Part model, mm, in its own coordinate system. A direction names the side the tool comes from. Coordinates: 2 decimals unless noted, no trailing zeros. Loops run counter-clockwise (first coordinate to the right, second up) from the corner with the lowest first, then second, coordinate; pieces in that order, holes last. Notation, with made-up numbers: (-20.75, 55.25) - (4.25, 55.25) arc R10 cw to (4.25, 71.25) - close; hole circle Ø8 at (34.25, 40.5). An arc over 180 degrees is marked (long way). Answer as CSV lines item,"result".
from build123d import *

# Parameters (mm, degrees)
F1_DEPTH = 60
F2_R     = 1.5
F3_DEPTH = 25
F4_W     = 70
F4_H     = 35
F5_DEPTH = 25
F6_R     = 5


with BuildPart() as f1:
    # F0 (on Front) → F1 (new body)
    with BuildSketch(Plane.XZ):
        Polygon((0, 6.5), (0, 0), (0, -3), (3, -3), (92.5, -3), (92.5, 0), (92.5, 6.395918), (89.5, 5.27192), (89.5, 4.5), (90.5, 4.5), (90.5, 0), (2, 0), (2, 4.5), (3, 4.5), (3, 6.5), align=None)
    extrude(amount=F1_DEPTH)

    # F2 (on face) → F3 (cut)
    with BuildSketch(Plane.XY):
        with Locations((45, -56.5)):
            Circle(F2_R)
        with Locations((44.5, -3.502359)):
            Circle(F2_R)
    extrude(amount=-F3_DEPTH, mode=Mode.SUBTRACT)

    # F4 (on face) → F5 (cut)
    with BuildSketch(Plane.XY):
        with Locations((46.2, -30)):
            Rectangle(F4_W, F4_H)
    extrude(amount=-F5_DEPTH, mode=Mode.SUBTRACT)

    # F6
    f6_edges = [f1.edges().sort_by_distance(p)[0] for p in [
        (11.2, -12.5, -1.5),
        (81.2, -47.5, -1.5),
        (81.2, -12.5, -1.5),
        (11.2, -47.5, -1.5),
    ]]
    fillet(f6_edges, radius=F6_R)


solid = f1.part
Q1. Which spindle directions (+Z, -Z, +X, -X, +Y, -Y) get a long thin tool onto all of the face, cutting with end or side? Do faces 1 (the face through (2, -30, 2)), 2 (the face through (12.7, -13.93, -1.52)), 3 (the face through (46, -50, -3)). Say none if no direction does.
Results:
face 1,"+Y, -Y"
face 2,"+Z, -Z"
face 3,"-Z, +X, -X, +Y, -Y"
Q2. Wall check: L1, parallel to X at y = -7, z = 0.75; L2, parallel to X at y = -48, z = 4.75; L3, parallel to Y at x = 45, z = -1.65. Give the ranges that are in metal, low to high.
Results:
L1,"x = 0 to 2, 90.5 to 92.5"
L2,"x = 0 to 3, 89.5 to 92.5"
L3,"y = -60 to -58, -55 to -47.5, -12.5 to -4.92, -2.09 to 0"
Q3. Saw through at B-B (y = -56.5). Give the cut face in (x, z).
Results:
outline,"(0, -3) - (43.5, -3) - (43.5, 0) - (2, 0) - (2, 4.5) - (3, 4.5) - (3, 6.5) - (0, 6.5) - close; (46.5, -3) - (92.5, -3) - (92.5, 6.4) - (89.5, 5.27) - (89.5, 4.5) - (90.5, 4.5) - (90.5, 0) - (46.5, 0) - close"
Q4. Saw through at A-A (x = 57.5). Give the cut face in (y, z).
Results:
outline,"(-60, -3) - (-47.5, -3) - (-47.5, 0) - (-60, 0) - close; (-12.5, -3) - (0, -3) - (0, 0) - (-12.5, 0) - close"
Q5. Saw through at D-D (x = 45). Give the cut face in (y, z), then the cut area to 3 significant figures.
Results:
outline,"(-60, -3) - (-58, -3) - (-58, 0) - (-60, 0) - close; (-55, -3) - (-47.5, -3) - (-47.5, 0) - (-55, 0) - close; (-12.5, -3) - (-4.92, -3) - (-4.92, 0) - (-12.5, 0) - close; (-2.09, -3) - (0, -3) - (0, 0) - (-2.09, 0) - close"
area,"57.5 mm^2"
Q6. Flat gauge pins, fed straight in: pin 1 (2 mm diameter, centred on y = -29, z = 2.5, fed in from -X); pin 2 (8 mm diameter, centred on x = 13, y = -22, fed in from +Z); pin 3 (1.8 mm diameter, centred on x = 44.5, y = -3.5, fed in from +Z). Where does each tip first touch, or does it go through?
Results:
pin 1,"stops at x = 0"
pin 2,"stops at z = 0"
pin 3,"passes through"
Q7. Two-plate mould, pull along Z, no slides. Class faces 4 (the face through (3, -30, 5)), 5 (the face through (90.5, -30, 2)), 6 (the face through (91.02, -29.58, 5.84)): released by +Z, released by -Z, zero draft, split by the parting line, or undercut.
Results:
face 4,"zero draft"
face 5,"undercut"
face 6,"released by +Z"
Q8. Saw through at C-C (z = 2). Give the cut face in (x, y).
Results:
outline,"(0, -60) - (2, -60) - (2, 0) - (0, 0) - close; (90.5, -60) - (92.5, -60) - (92.5, 0) - (90.5, 0) - close"
